For this review, use the dimensioned drawing (mm, ordinates from the lowest corner) and the shaded views. A direction names the side the tool comes from. Coordinates: 2 decimals unless noted, no trailing zeros. Order: outer loops, then holes, each group sorted by start corner. A loop starts at its lowest first (then second) coordinate and runs counter-clockwise, first axis right, second up. Notation, with made-up numbers: M -2,86 L 24,86 A17 ccw 24,96 Z; hole C 2,-4 d3. An arc over 180 degrees is marked long. Answer in a Markdown table with one row per item.
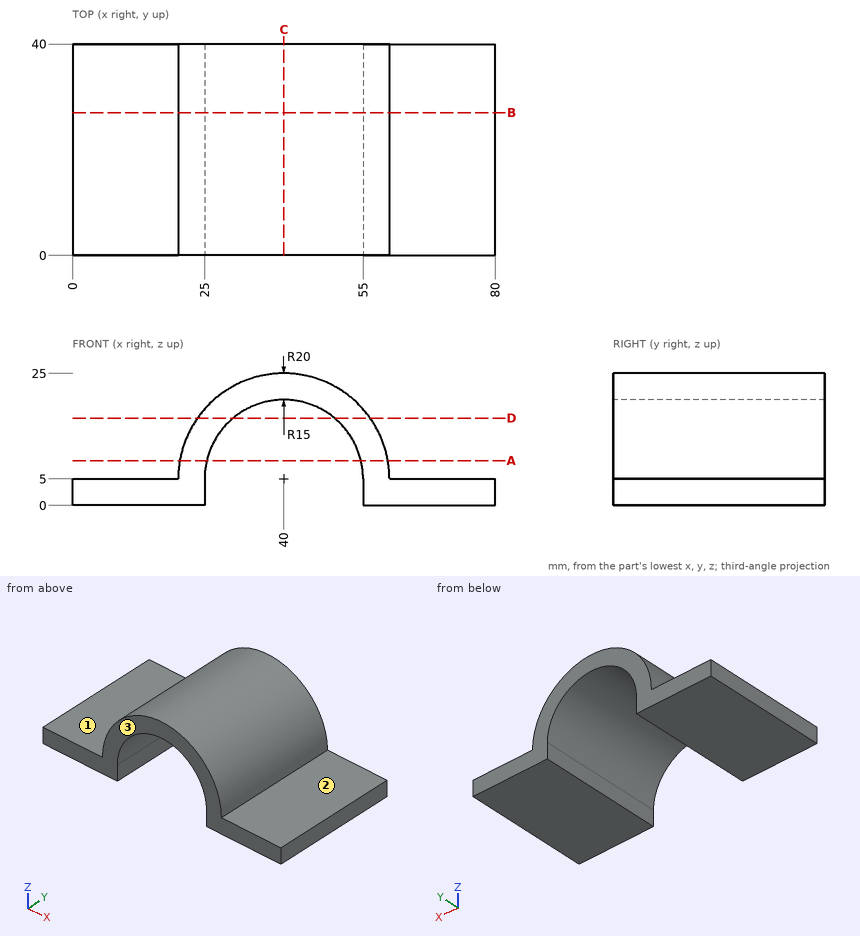
(1) Add section D-D, the plane z = 16.5. Give the boundary of the cut face in (x, y), and give its area (3 significant figures).
Return value:
| item | result |
|---|---|
| outline | M 23.64,0 L 30.37,0 L 30.37,40 L 23.64,40 Z; M 49.63,0 L 56.36,0 L 56.36,40 L 49.63,40 Z |
| area | 539 mm2 |
(2) Add section A-A, the plane z = 8.5. Give the boundary of the cut face in (x, y).
Return value:
| item | result |
|---|---|
| outline | M 20.31,0 L 25.41,0 L 25.41,40 L 20.31,40 Z; M 54.59,0 L 59.69,0 L 59.69,40 L 54.59,40 Z |
(3) For line 1 along X through (y, z) = (11.5, 2.5); line 2 along X through (y, z) = (32, 9.5); line 3 along Z through (x, y) = (9, 26.5), list the stretches that pass through material, from the lowest coordinate up. Write a range as from..to.
Return value:
| item | result |
|---|---|
| line 1 | x = 0..25, 55..80 |
| line 2 | x = 20.51..25.69, 54.31..59.49 |
| line 3 | z = 0..5 |
(4) For the marked faces 1, 2 and 3, list the 3-axis set-ups (+Z, -Z, +X, -X, +Y, -Y) from which the entire face can be reached by the end or side of a thin tool; tool diameter is ignored.
Return value:
| item | result |
|---|---|
| face 1 | +Z, -X, +Y, -Y |
| face 2 | +Z, +X, +Y, -Y |
| face 3 | +Z, -Z, +X, -X, -Y |
(5) Add section C-C, the plane x = 40. Give the boundary of the cut face in (y, z), and give its area (3 significant figures).
Return value:
| item | result |
|---|---|
| outline | M 0,20 L 40,20 L 40,25 L 0,25 Z |
| area | 200 mm2 |
(6) Add section B-B, the plane y = 27. Give the boundary of the cut face in (x, z).
Return value:
| item | result |
|---|---|
| outline | M 0,0 L 25,0 L 25,5 A15 cw 55,5 L 55,0 L 80,0 L 80,5 L 60,5 A20 ccw 20,5 L 0,5 Z |
(7) Insertion check: pin 1 Ø22 at (x, y) = (73, 17.5) entering from +Z; pin 2 Ø1.5 at (x, y) = (37, 8.5) entering from -Z; pin 3 Ø10 at (x, y) = (39, 9) entering from -Z; pin 4 Ø1.5 at (x, z) = (27.5, 6) entering from +Y. Each pin has a flat end and moves straight along its axis. Give the tip position at first contact, or say it passes through.
Return value:
| item | result |
|---|---|
| pin 1 | stops at z = 5 |
| pin 2 | stops at z = 19.52 |
| pin 3 | stops at z = 18.75 |
| pin 4 | passes through |
